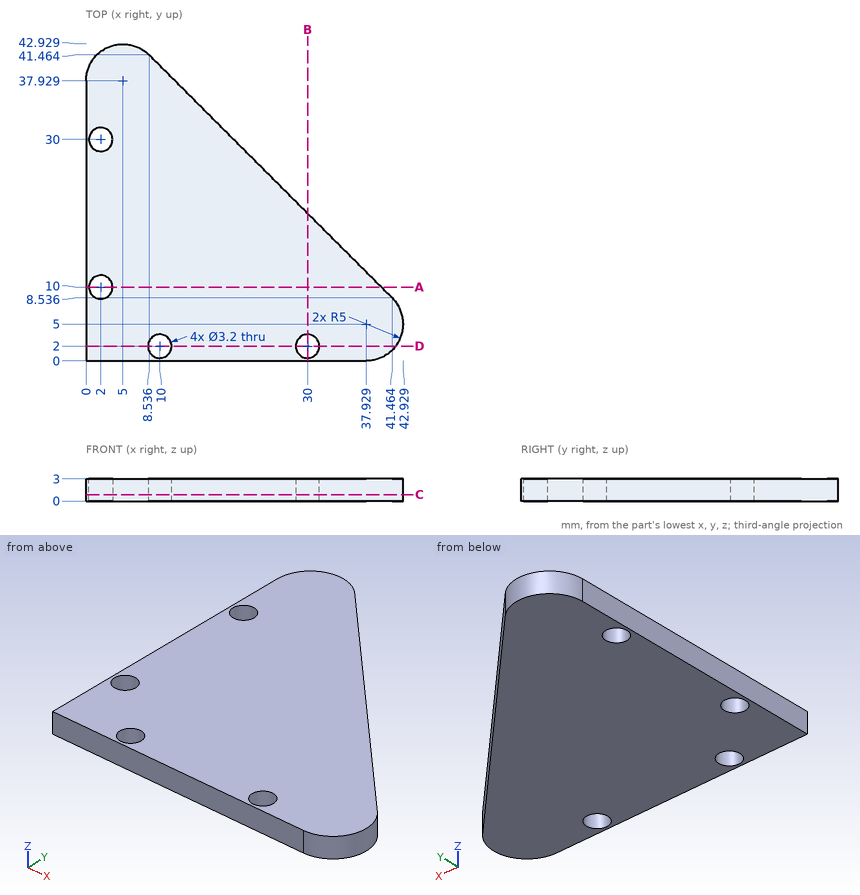
Print and shaded views of the part. All mm, measured from the part's lowest x, y and z. Coordinates: 2 decimals unless noted, no trailing zeros. Loops run counter-clockwise (first coordinate to the right, second up) from the corner with the lowest first, then second, coordinate; pieces in that order, holes last. Notation, with made-up numbers: (22.25, 51.5) -> (73.25, 51.5) arc R24 cw to (73.25, 89.5) -> close; hole circle Ø9 at (58, 1). An arc over 180 degrees is marked (long way). Use a Markdown table: item, result. Add a question column.
Item 1: Band-saw the part on C-C on z = 0.9. Write the cut outline in (x, y) (1 decimal).
Item 2: Band-saw the part on D-D on y = 2. Write the cut outline in (x, z).
Item 3: Band-saw the part on A-A on y = 10. Write the cut outline in (x, z).
Item 4: Flat gauge pins, fed straight in: P1, Ø1.5, axis at y = 28, z = 0.5, coming from the +X side; P2, Ø5, axis at x = 2, y = 30, coming from the -Z side; P3, Ø1.9, axis at x = 2, y = 10, coming from the +Z side; P4, Ø1.5, axis at x = 38.5, z = 1.5, coming from the +Y side. Where does each tip first touch, or does it go through?
Item 5: Band-saw the part on B-B on x = 30. Write the cut outline in (y, z), plus the area to 3 significant figures.
Item 6: Probe probe 1 along Y at (x, z) = (2, 0.95); probe 2 along Y at (x, z) = (29.5, 1.65); probe 3 along X at (y, z) = (9, 0.85). List the from-to ranges inside material, lowest first.
Geometry says:
| question | item | result |
|---|---|---|
| 1 | outline | (0, 0) -> (37.9, 0) arc R5 ccw to (41.5, 8.5) -> (8.5, 41.5) arc R5 ccw to (0, 37.9) -> close; hole circle Ø3.2 at (2, 10); hole circle Ø3.2 at (2, 30); hole circle Ø3.2 at (10, 2); hole circle Ø3.2 at (30, 2) |
| 2 | outline | (0, 0) -> (8.4, 0) -> (8.4, 3) -> (0, 3) -> close; (11.6, 0) -> (28.4, 0) -> (28.4, 3) -> (11.6, 3) -> close; (31.6, 0) -> (41.93, 0) -> (41.93, 3) -> (31.6, 3) -> close |
| 3 | outline | (0, 0) -> (0.4, 0) -> (0.4, 3) -> (0, 3) -> close; (3.6, 0) -> (40, 0) -> (40, 3) -> (3.6, 3) -> close |
| 4 | P1 | x = 22.75 |
| 4 | P2 | z = 0 |
| 4 | P3 | through |
| 4 | P4 | y = 12.25 |
| 5 | outline | (0, 0) -> (0.4, 0) -> (0.4, 3) -> (0, 3) -> close; (3.6, 0) -> (20, 0) -> (20, 3) -> (3.6, 3) -> close |
| 5 | area | 50.4 mm² |
| 6 | probe 1 | 0 to 8.4, 11.6 to 28.4, 31.6 to 41.93 |
| 6 | probe 2 | 0 to 0.48, 3.52 to 20.5 |
| 6 | probe 3 | 0 to 0.75, 3.25 to 41 |
